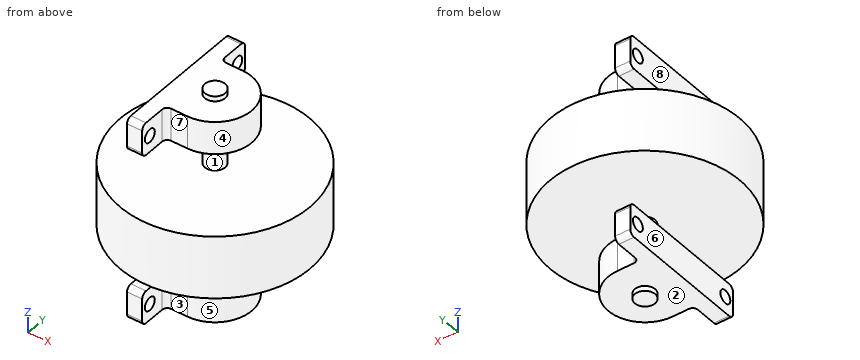
```python
from build123d import *

# Parameters (mm, degrees)
SKETCH_1_R           = 37.5
EXTRUDE_1_DEPTH      = 12.5
EXTRUDE_1_DEPTH_BACK = 12.5
SKETCH_1_3_R         = 4
EXTRUDE_2_DEPTH      = 42.5
EXTRUDE_2_DEPTH_BACK = 42.5
SKETCH_2_R           = 14.5
SKETCH_2_W           = 14.5
SKETCH_2_H           = 29
SKETCH_2_W_2         = 6
SKETCH_2_H_2         = 54
EXTRUDE_3_DEPTH      = 13
SKETCH_3_R           = 14.5
SKETCH_3_W           = 14.5
SKETCH_3_H           = 29
SKETCH_3_W_2         = 6
SKETCH_3_H_2         = 54
EXTRUDE_4_DEPTH      = 13
SKETCH_4_R           = 2.6
CUT_EXTRUDE_1_DEPTH  = 30
FILLET_1_R           = 2


with BuildPart() as part:
    # Sketch 1 → Extrude 1 (new body, two sides)
    with BuildSketch(Plane.XY) as extrude_1_sk:
        Circle(SKETCH_1_R)
    extrude(amount=EXTRUDE_1_DEPTH)
    extrude(extrude_1_sk.sketch, amount=-EXTRUDE_1_DEPTH_BACK)

    # Sketch 1_3 → Extrude 2 (add, two sides)
    with BuildSketch(Plane.XY) as extrude_2_sk:
        Circle(SKETCH_1_3_R)
    extrude(amount=EXTRUDE_2_DEPTH)
    extrude(extrude_2_sk.sketch, amount=-EXTRUDE_2_DEPTH_BACK)

    # Sketch 2 → Extrude 3 (add)
    with BuildSketch(Plane.XY.offset(40.5)):
        Circle(SKETCH_2_R)
        with Locations((-7.25, 0)):
            Rectangle(SKETCH_2_W, SKETCH_2_H)
        with Locations((-11.5, 0)):
            Rectangle(SKETCH_2_W_2, SKETCH_2_H_2)
    extrude(amount=-EXTRUDE_3_DEPTH)

    # Sketch 3 → Extrude 4 (add)
    with BuildSketch(Plane(origin=(0, 0, -40.5), x_dir=(-1, 0, 0), z_dir=(0, 0, -1))):
        Circle(SKETCH_3_R)
        with Locations((7.25, 0)):
            Rectangle(SKETCH_3_W, SKETCH_3_H)
        with Locations((11.5, 0)):
            Rectangle(SKETCH_3_W_2, SKETCH_3_H_2)
    extrude(amount=-EXTRUDE_4_DEPTH)

    # Sketch 4 → Cut-Extrude 1 (cut, through all)
    with BuildSketch(Plane(origin=(-8.5, 0, 0), x_dir=(0, 0, -1), z_dir=(1, 0, 0))):
        with Locations((34, 23)):
            Circle(SKETCH_4_R)
        with Locations((34, -23)):
            Circle(SKETCH_4_R)
        with Locations((-34, -23)):
            Circle(SKETCH_4_R)
        with Locations((-34, 23)):
            Circle(SKETCH_4_R)
    extrude(amount=-CUT_EXTRUDE_1_DEPTH, mode=Mode.SUBTRACT)

    # Fillet 1
    fillet_1_edges = [part.edges().sort_by_distance(p)[0] for p in [
        (-11.5, 27, 40.5),
        (-11.5, -27, 27.5),
        (-11.5, 27, 27.5),
        (-8.5, 14.5, 34),
        (-8.5, -14.5, 34),
        (-11.5, -27, 40.5),
        (-11.5, -27, -40.5),
        (-11.5, 27, -27.5),
        (-11.5, -27, -27.5),
        (-8.5, -14.5, -34),
        (-8.5, 14.5, -34),
        (-11.5, 27, -40.5),
    ]]
    fillet(fillet_1_edges, radius=FILLET_1_R)


solid = part.part
```
CAD build for the part. Positions are in the model's coordinates, mm. Face numbers are marked on the shaded views. A direction names the side the tool comes from. Round coordinates to 2 decimals unless told otherwise and drop trailing zeros. Loops run counter-clockwise (first coordinate to the right, second up) from the corner with the lowest first, then second, coordinate; pieces in that order, holes last. Notation, with made-up numbers: M 45.25,30 L 68.25,30 A12 cw 68.25,35 Z; hole C 31,45.25 d2. An arc over 180 degrees is marked long. Use a Markdown table: item, result. Add a question column.
(1) Flat gauge pins, fed straight in: pin 1 (5 mm diameter, centred on x = -2, z = 36, fed in from +Y); pin 2 (1 mm diameter, centred on x = -3.5, y = 16, fed in from +Z); pin 3 (6 mm diameter, centred on x = -14.5, z = -13, fed in from +Y); pin 4 (23 mm diameter, centred on x = -5, y = 5.5, fed in from +Z). Where does each tip first touch, or does it go through?
(2) Cut at C-C (y = -23). Give the cut face in (x, z), and give its area (3 significant figures).
(3) Which spindle directions (+Z, -Z, +X, -X, +Y, -Y) get a long thin tool onto all of the face, cutting with end or side? Do the marked faces 4, 5, 6, 7 and 8. Say none if no direction does.
(4) Pull direction Z, two halves, no side cores. Call the marked faces 1, 2 and 3: +Z half, -Z half, draft (parallel to the pull), parting line (faces both ways), or undercut.
(5) Drill centre lines: line 1 (Y direction, x = -12.5, z = -34); line 2 (Z direction, x = 14, y = 2); line 3 (Z direction, x = -26, y = -10). Where is each one in solid material? Low to high.
(6) Cut at B-B (z = 34). Give the cut face in (x, y), and give its area (3 significant figures).
(7) Cut at A-A (x = -12.5). Give the cut face in (y, z), and give its area (3 significant figures).
(8) Cut at D-D (y = 0). Give the cut face in (x, z), and give its area (3 significant figures).
Geometry says:
| question | item | result |
|---|---|---|
| 1 | pin 1 | stops at y = 14.5 |
| 1 | pin 2 | stops at z = 12.5 |
| 1 | pin 3 | stops at y = 35.68 |
| 1 | pin 4 | stops at z = 42.5 |
| 2 | outline | M -29.62,-12.5 L 29.62,-12.5 L 29.62,12.5 L -29.62,12.5 Z; M -14.5,-40.5 L -8.5,-40.5 L -8.5,-36.6 L -14.5,-36.6 Z; M -14.5,-31.4 L -8.5,-31.4 L -8.5,-27.5 L -14.5,-27.5 Z; M -14.5,27.5 L -8.5,27.5 L -8.5,31.4 L -14.5,31.4 Z; M -14.5,36.6 L -8.5,36.6 L -8.5,40.5 L -14.5,40.5 Z |
| 2 | area | 1,570 mm² |
| 3 | face 4 | +Z, +X |
| 3 | face 5 | -Z, +X |
| 3 | face 6 | -Z, -X, +Y, -Y |
| 3 | face 7 | +Z, +X, -Y |
| 3 | face 8 | +Z, -X, +Y, -Y |
| 4 | face 1 | undercut |
| 4 | face 2 | -Z half |
| 4 | face 3 | draft |
| 5 | line 1 | y = -27 to -25.6, -20.4 to 20.4, 25.6 to 27 |
| 5 | line 2 | z = -40.5 to -27.5, -12.5 to 12.5, 27.5 to 40.5 |
| 5 | line 3 | z = -12.5 to 12.5 |
| 6 | outline | M -14.5,-27 L -8.5,-27 L -8.5,-25.6 L -14.5,-25.6 Z; M -14.5,-20.4 L -8.5,-20.4 L -8.5,-16.5 A2 cw -6.5,-14.5 L 0,-14.5 A14.5 ccw 0,14.5 L -6.5,14.5 A2 cw -8.5,16.5 L -8.5,20.4 L -14.5,20.4 Z; M -14.5,25.6 L -8.5,25.6 L -8.5,27 L -14.5,27 Z |
| 6 | area | 840 mm² |
| 7 | outline | M -35.36,-12.5 L 35.36,-12.5 L 35.36,12.5 L -35.36,12.5 Z; M -27,-38.5 A2 ccw -25,-40.5 L 25,-40.5 A2 ccw 27,-38.5 L 27,-29.5 A2 ccw 25,-27.5 L -25,-27.5 A2 ccw -27,-29.5 Z; M -27,29.5 A2 ccw -25,27.5 L 25,27.5 A2 ccw 27,29.5 L 27,38.5 A2 ccw 25,40.5 L -25,40.5 A2 ccw -27,38.5 Z; hole C -23,-34 d5.2; hole C -23,34 d5.2; hole C 23,-34 d5.2; hole C 23,34 d5.2 |
| 7 | area | 3,080 mm² |
| 8 | outline | M -37.5,-12.5 L -4,-12.5 L -4,-27.5 L -14.5,-27.5 L -14.5,-40.5 L -4,-40.5 L -4,-42.5 L 4,-42.5 L 4,-40.5 L 14.5,-40.5 L 14.5,-27.5 L 4,-27.5 L 4,-12.5 L 37.5,-12.5 L 37.5,12.5 L 4,12.5 L 4,27.5 L 14.5,27.5 L 14.5,40.5 L 4,40.5 L 4,42.5 L -4,42.5 L -4,40.5 L -14.5,40.5 L -14.5,27.5 L -4,27.5 L -4,12.5 L -37.5,12.5 Z |
| 8 | area | 2,900 mm² |
